For this review, take the finished solid that the model builds, in its own axes (mm). Face numbers are marked on the shaded views. A direction names the side the tool comes from. Coordinates: 2 decimals unless noted, no trailing zeros. Write each loop counter-clockwise with the first axis right and the second up, starting at its lowest first coordinate (ties: lowest second). Pieces come first, ordered by that corner, then holes. Notation, with made-up numbers: (40, 63.5) -> (62, 63.5) arc R16 ccw to (62, 81.5) -> close; hole circle Ø11 at (-6, -5.75). An arc over 180 degrees is marked (long way). Put each result on its own line as item: value. Start each with the question number.
Item 1: For the marked faces 1 and 2, list the 3-axis set-ups (+Z, -Z, +X, -X, +Y, -Y) from which the entire face can be reached by the end or side of a thin tool; tool diameter is ignored.
Item 2: The part is to be moulded in two halves that separate along Y. For the marked faces 3, 4, 5 and 6, say which applies: +Y half, -Y half, draft (parallel to the pull), parting line (faces both ways), or undercut.
Item 3: Consider section B-B on x = 12.7. Give the boundary of the cut face in (y, z).
Item 4: Consider section D-D on y = -2.25. Give the boundary of the cut face in (x, z), and give its area (3 significant figures).
Item 5: Insertion check: P1, Ø2, axis at x = 5, z = 1.5, coming from the +Y side; P2, Ø1, axis at x = 6.5, z = 1, coming from the +Y side. Each pin has a flat end and moves straight along its axis. Give the tip position at first contact, or say it passes through.
Item 6: Consider section C-C on z = 1.2. Give the boundary of the cut face in (x, y).
Item 7: Consider section A-A on y = 0. Give the boundary of the cut face in (x, z).
Item 8: To check wall thickness, follow L1, parallel to X at y = 1.25, z = 3.75; L2, parallel to Z at x = 7.5, y = 2.5; L3, parallel to X at y = -1, z = 0.7. State the ranges of each line that lie inside material, in increasing order.
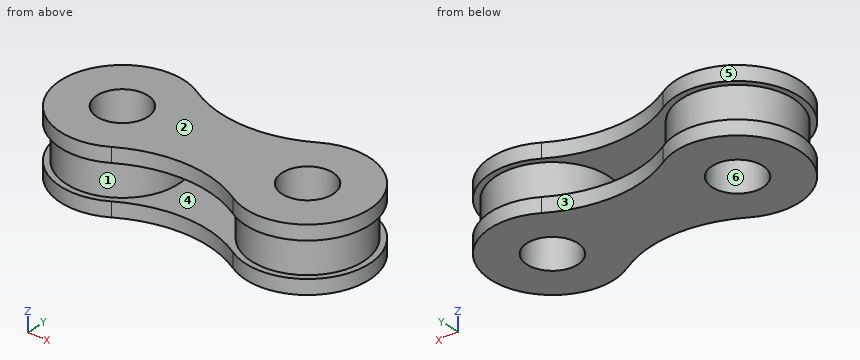
```python
from build123d import *

# Parameters (mm, degrees)
SKETCH1_R           = 1.75
BOSS_EXTRUDE1_DEPTH = 1
BOSS_EXTRUDE3_REACH = 19.802
SKETCH4_R           = 3.85
SKETCH4_R_2         = 1.75


with BuildPart() as part:
    # Sketch1 → Boss-Extrude1 (new body)
    with BuildSketch(Plane.XY):
        with BuildLine():
            ThreePointArc((2.177163766, 3.649994238), (-4.25, 0), (2.177163766, -3.649994238))
            ThreePointArc((2.177163766, -3.649994238), (6.35, -2.5), (10.522836234, -3.649994238))
            ThreePointArc((10.522836234, -3.649994238), (16.95, 0), (10.522836234, 3.649994238))
            ThreePointArc((10.522836234, 3.649994238), (6.35, 2.5), (2.177163766, 3.649994238))
        make_face()
        Circle(SKETCH1_R, mode=Mode.SUBTRACT)
        with Locations((12.7, 0)):
            Circle(SKETCH1_R, mode=Mode.SUBTRACT)
    extrude(amount=BOSS_EXTRUDE1_DEPTH)


with BuildPart() as body_2:
    # Body-Move_Copy1: copy of part
    add(part.part.moved(Location((0, 0, 3.4))))

    # Sketch4 → Boss-Extrude3 (add, up to next)
    with BuildSketch(Plane.XY.offset(1), mode=Mode.PRIVATE) as boss_extrude3_sk1:
        with Locations(Location((0, 0, 0), (0, 0, 180))):
            Circle(SKETCH4_R)
        Circle(SKETCH4_R_2, mode=Mode.SUBTRACT)
    boss_extrude3_tool1 = extrude(boss_extrude3_sk1.sketch, amount=BOSS_EXTRUDE3_REACH, mode=Mode.PRIVATE) - body_2.part
    # Sketch4 → Boss-Extrude3 (add, up to next)
    with BuildSketch(Plane.XY.offset(1), mode=Mode.PRIVATE) as boss_extrude3_sk2:
        with Locations(Location((12.7, 0, 0), (0, 0, 180))):
            Circle(SKETCH4_R)
        with Locations((12.7, 0)):
            Circle(SKETCH4_R_2, mode=Mode.SUBTRACT)
    boss_extrude3_tool2 = extrude(boss_extrude3_sk2.sketch, amount=BOSS_EXTRUDE3_REACH, mode=Mode.PRIVATE) - body_2.part

    add(part.part)  # Boss-Extrude3 merges part
    add(boss_extrude3_tool1.solids().sort_by_distance((3.741106, 0, 1))[0])
    add(boss_extrude3_tool2.solids().sort_by_distance((16.441106, 0, 1))[0])


solid = body_2.part
```
Return value:
1. face 1: none
1. face 2: +Z, +X, -X, +Y, -Y
2. face 3: +Y half
2. face 4: draft
2. face 5: parting line
2. face 6: undercut
3. outline: (-4.25, 0) -> (-1.75, 0) -> (-1.75, 4.4) -> (-4.25, 4.4) -> (-4.25, 3.4) -> (-3.85, 3.4) -> (-3.85, 1) -> (-4.25, 1) -> close; (1.75, 0) -> (4.25, 0) -> (4.25, 1) -> (3.85, 1) -> (3.85, 3.4) -> (4.25, 3.4) -> (4.25, 4.4) -> (1.75, 4.4) -> close
4. outline: (-3.61, 0) -> (16.31, 0) -> (16.31, 1) -> (15.82, 1) -> (15.82, 3.4) -> (16.31, 3.4) -> (16.31, 4.4) -> (-3.61, 4.4) -> (-3.61, 3.4) -> (-3.12, 3.4) -> (-3.12, 1) -> (-3.61, 1) -> close; hole (3.12, 1) -> (9.58, 1) -> (9.58, 3.4) -> (3.12, 3.4) -> close
4. area: 69.8 mm^2
5. P1: y = 2.81
5. P2: y = 2.53
6. outline: circle Ø7.7 at (0, 0); circle Ø7.7 at (12.7, 0); hole circle Ø3.5 at (0, 0); hole circle Ø3.5 at (12.7, 0)
7. outline: (-4.25, 0) -> (-1.75, 0) -> (-1.75, 4.4) -> (-4.25, 4.4) -> (-4.25, 3.4) -> (-3.85, 3.4) -> (-3.85, 1) -> (-4.25, 1) -> close; (1.75, 0) -> (10.95, 0) -> (10.95, 4.4) -> (1.75, 4.4) -> close; (14.45, 0) -> (16.95, 0) -> (16.95, 1) -> (16.55, 1) -> (16.55, 3.4) -> (16.95, 3.4) -> (16.95, 4.4) -> (14.45, 4.4) -> close; hole (3.85, 1) -> (8.85, 1) -> (8.85, 3.4) -> (3.85, 3.4) -> close
8. L1: -4.06 to -1.22, 1.22 to 11.48, 13.92 to 16.76
8. L2: 0 to 1, 3.4 to 4.4
8. L3: -4.13 to -1.44, 1.44 to 11.26, 14.14 to 16.83
